Answer from the drawing. Dimensions are ordinates in mm from the lowest x, y and z of the part. Give positions to 0.01 mm unless a question says otherwise; leave off trailing zeros. Loops run counter-clockwise (first coordinate to the right, second up) from the corner with the lowest first, then second, coordinate; pieces in that order, holes last. Notation, with made-up numbers: (-37, -36) -> (-21, -36) arc R17 ccw to (-21, -26) -> close; hole circle Ø4 at (29, -32). An arc over 180 degrees is marked (long way). Write each question's results on one line, items separated by ' | '. Start each with the question number.
Item 1: Find the intervals of material crossed by line 1 (Z direction, x = 17.5, y = 8.5); line 2 (X direction, y = 11.75, z = 30); line 3 (X direction, y = 11.75, z = 35), in increasing order.
Item 2: Section A-A on z = 30 is taken. Write down the section's boundary in (x, y), and give its area (3 significant figures).
Item 3: Determine the mould class of the marked faces 1, 2 and 3 for opening direction X: +X half, -X half, draft (parallel to the pull), parting line (faces both ways), or undercut.
Item 4: Section C-C on y = 18.5 is taken. Write down the section's boundary in (x, z), and give its area (3 significant figures).
Item 5: Each of these flat-tipped pins is pushed along its axis until it touches: P1, Ø10, axis at x = 30.5, z = 11.5, coming from the -Y side; P2, Ø20.5, axis at x = 17.5, z = 30, coming from the +Y side. Where does it stop, or does it pass through?
Item 6: Section B-B on x = 17.5 is taken. Write down the section's boundary in (y, z), and give its area (3 significant figures).
Item 7: Section D-D on x = 2 is taken. Write down the section's boundary in (y, z), and give its area (3 significant figures).
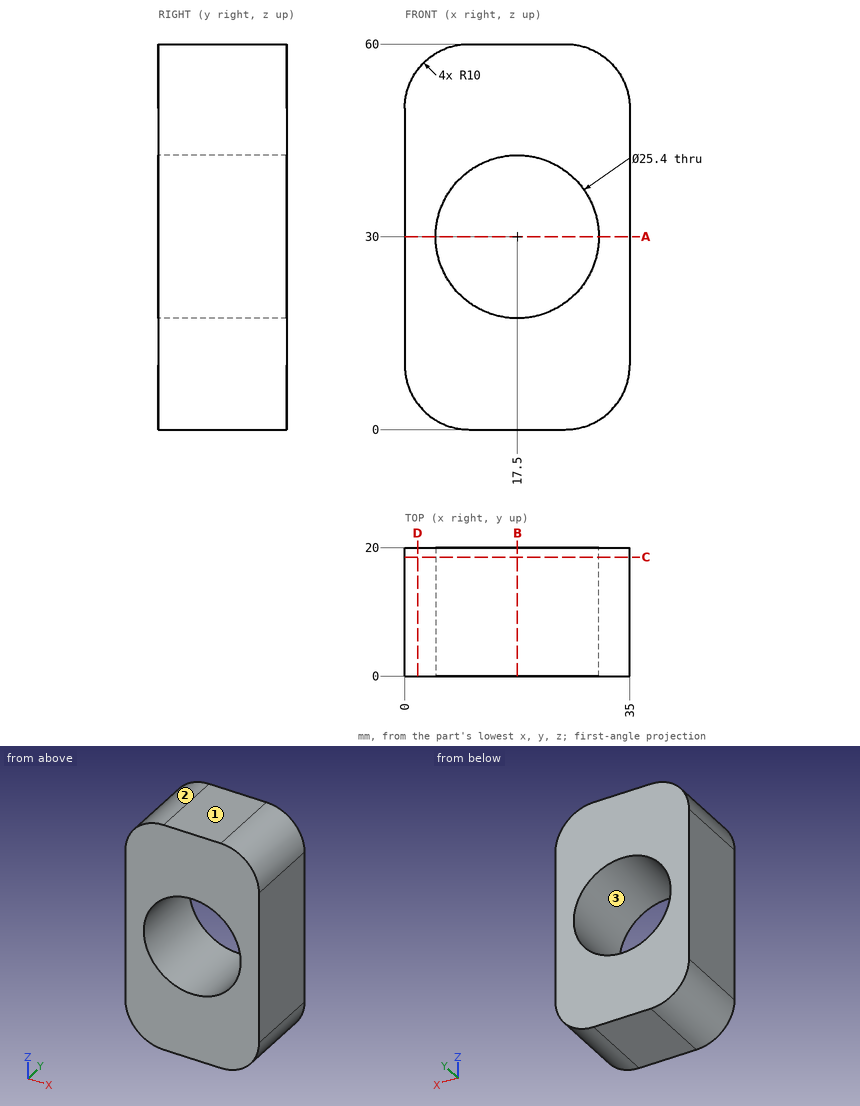
Findings:
1) line 1: 0 to 17.3, 42.7 to 60 | line 2: 0 to 4.8, 30.2 to 35 | line 3: 0 to 5.83, 29.17 to 35
2) outline: (0, 0) -> (4.8, 0) -> (4.8, 20) -> (0, 20) -> close; (30.2, 0) -> (35, 0) -> (35, 20) -> (30.2, 20) -> close | area: 192 mm2
3) face 1: draft | face 2: -X half | face 3: undercut
4) outline: (0, 10) arc R10 ccw to (10, 0) -> (25, 0) arc R10 ccw to (35, 10) -> (35, 50) arc R10 ccw to (25, 60) -> (10, 60) arc R10 ccw to (0, 50) -> close; hole circle Ø25.4 at (17.5, 30) | area: 1,510 mm2
5) P1: y = 0 | P2: through
6) outline: (0, 0) -> (20, 0) -> (20, 17.3) -> (0, 17.3) -> close; (0, 42.7) -> (20, 42.7) -> (20, 60) -> (0, 60) -> close | area: 692 mm2
7) outline: (0, 4) -> (20, 4) -> (20, 56) -> (0, 56) -> close | area: 1,040 mm2
